Read the model definition and answer for the solid it produces. Units are mm, in the model's axes. A direction names the side the tool comes from. Coordinates: 2 decimals unless noted, no trailing zeros. Loops run counter-clockwise (first coordinate to the right, second up) from the corner with the lowest first, then second, coordinate; pieces in that order, holes last. Notation, with made-up numbers: M 57,11.5 L 108,11.5 A20 ccw 108,42.5 Z; hole C -33,77 d6. An arc over 180 degrees is marked long. Use one line per item in the form item = value. Start each with the question number.
1. The part is cut by section A-A (x = 4.5). Give the vertices of the cut face in (y, z).
2. The part is cut by section D-D (y = 26.2). Give the vertices of the cut face in (x, z), plus the area to 4 significant figures.
3. For a pull along X with two mould halves and no side action, classify faces 4 (the flat face through (11.59, -2.66, 1.48)), 5 (the flat face through (6, 17, 0)), 6 (the cylindrical face through (4.05, 43.83, 1.52)), 7 (the cylindrical face through (5.4, 56.2, 1.5)) as released by +X, released by -X, zero draft, split by the parting line, or undercut.
4. The part is cut by section C-C (z = 1.85). Give the number of separate pieces and of enclosed holes in the cut face, plus the area to 3 significant figures.
5. The part is cut by section B-B (y = 57.4). Give the vertices of the cut face in (x, z).
6. Find the intervals of material crossed by probe 1 along Y at (x, z) = (4.5, 1.05); probe 2 along X at (y, z) = (42.4, 2.1); probe 3 along Y at (x, z) = (9.75, 0.7), in increasing order. Write a range as [from, to].
7. A tool of negligible diameter and unlimited length cuts with its end or side. For faces 1 (the flat face through (9, 49, 1)), 2 (the flat face through (9, -16, 1)), 3 (the flat face through (15.75, 16, 1)), from which of +Z, -Z, +X, -X, +Y, -Y can it reach the whole face along a straight path? Write none if from no direction.
8. Flat-ended cylindrical pins translate along their axes: pin 1 (3.5 mm diameter, centred on x = 4.5, y = 42.4, fed in from -Z); pin 2 (1.5 mm diameter, centred on x = 10.5, z = 1.5, fed in from -Y). Find the tip coordinate at first contact, or state that the pin passes through.
Autodesk Inventor part; units mm, degrees
ref_plane "YZ Plane" through (0, 0, 0) normal (1, 0, 0) x (0, 1, 0)
ref_plane "XZ Plane" through (0, 0, 0) normal (0, 1, 0) x (-1, 0, 0)
ref_plane "XY Plane" through (0, 0, 0) normal (0, 0, 1) x (1, 0, 0)
sketch "Szkic1" plane through (0, 0, 0) normal (0, 0, 1) x (1, 0, 0)
  line L0 (0, 0) -> (15.75, 0)
  line L1 (15.75, 0) -> (15.75, 32.4)
  line L2 (0, 32.4) -> (15.75, 32.4)
  line L3 (0, 0) -> (0, 32.4)
  line L4 (0, 0) -> (9, 0)
  line L5 (9, 0) -> (9, -30)
  line L6 (9, -30) -> (0, -30)
  line L7 (0, -30) -> (0, 0)
  line L8 (0, 32.4) -> (9, 32.4)
  line L9 (9, 32.4) -> (9, 62.4)
  line L10 (9, 62.4) -> (0, 62.4)
  line L11 (0, 62.4) -> (0, 32.4)
  point P0 (15.1556, 0)
  point P1 (9.75, 26.2)
  point P2 (9.75, 6.2)
  point P3 (4.5, -25)
  point P4 (4.5, -10)
  point P5 (4.5, 42.4)
  point P6 (4.5, 57.4)
  dimension "d0" = 9.75
  dimension "d1" = 9.75
  dimension "d2" = 6.2
  dimension "d3" = 6.2
  dimension "d13" = 15.75
  dimension "d14" = 32.4
  dimension "d18" = 9
  dimension "d19" = 30
  dimension "d20" = 9
  dimension "d21" = 30
  dimension "d31" = 4.5
  dimension "d32" = 4.5
  dimension "d33" = 4.5
  dimension "d34" = 4.5
  dimension "d35" = 5
  dimension "d36" = 5
  dimension "d37" = 15
  dimension "d38" = 15
extrude "Wyciągnięcie proste1" add sketch "Szkic1" along normal blind 3 contours L3 L2 L1 L0
hole "Otwór1" at (9.75, 6.2, 0) at (9.75, 26.2, 0) direction (0, 0, 1) diameter 3 end through all
chamfer "Faza1" distance 1.5 angle 45 2 edges at (15.75, 0, 1.5) (15.75, 32.4, 1.5)
extrude "Wyciągnięcie proste2" add sketch "Szkic1" along normal blind 3 contours L0 L5 L6 L7 | L11 L10 L9 L2
chamfer "Faza2" distance 5.25 distance2 5.25 1 edges at (9, 32.4, 1.5) measured on face at (12.5, 32.4, 1)
chamfer "Faza3" distance 5.25 distance2 5.25 1 edges at (9, 0, 1.5) measured on face at (10.75, 0, 1)
fillet "Zaokrąglenie1" radius 2 4 edges at (9, -30, 1.5) (0, -30, 1.5) (9, 62.4, 1.5) (0, 62.4, 1.5)
hole "Otwór2" at (4.5, -25, 0) at (4.5, -10, 0) at (4.5, 42.4, 0) at (4.5, 57.4, 0) direction (0, 0, 1) diameter 3 end through all
equation "\"d18\" = d20"
equation "\"d19\" = d21"
properties part number "LC_ALU_3mm_X_Axis_Carriage_Accesory_Mounting_Bracket"
Computed values:
q1.outline = M -30,0 L -26.5,0 L -26.5,3 L -30,3 Z; M -23.5,0 L -11.5,0 L -11.5,3 L -23.5,3 Z; M -8.5,0 L 40.9,0 L 40.9,3 L -8.5,3 Z; M 43.9,0 L 55.9,0 L 55.9,3 L 43.9,3 Z; M 58.9,0 L 62.4,0 L 62.4,3 L 58.9,3 Z
q2.outline = M 0,0 L 8.25,0 L 8.25,3 L 0,3 Z; M 11.25,0 L 15.75,0 L 15.75,3 L 11.25,3 Z
q2.area = 38.25 mm²
q3.face_4 = released by +X
q3.face_5 = zero draft
q3.face_6 = undercut
q3.face_7 = undercut
q4.separate_pieces = 1
q4.enclosed_holes = 6
q4.area = 1,030 mm²
q5.outline = M 0,0 L 3,0 L 3,3 L 0,3 Z; M 6,0 L 9,0 L 9,3 L 6,3 Z
q6.probe_1 = [-30, -26.5], [-23.5, -11.5], [-8.5, 40.9], [43.9, 55.9], [58.9, 62.4]
q6.probe_2 = [0, 3], [6, 9]
q6.probe_3 = [-4.5, 4.7], [7.7, 24.7], [27.7, 36.9]
q7.face_1 = +Z, -Z, +X, +Y
q7.face_2 = +Z, -Z, +X, -Y
q7.face_3 = +Z, -Z, +X, +Y, -Y
q8.pin_1 = 0
q8.pin_2 = -4.5
